Autodesk Inventor part; units mm, degrees
ref_plane "YZ Plane" through (0, 0, 0) normal (1, 0, 0) x (0, 1, 0)
ref_plane "XZ Plane" through (0, 0, 0) normal (0, 1, 0) x (-1, 0, 0)
ref_plane "XY Plane" through (0, 0, 0) normal (0, 0, 1) x (1, 0, 0)
sketch "草图1" plane through (0, 0, 0) normal (1, 0, 0) x (0, 1, 0)
  line L0 (-7.0511, 44.9164) -> (14.9489, 44.9164)
  line L1 (59.1261, -96.2836) -> (10.702, 41.9164)
  line L2 (10.702, 41.9164) -> (-7.0511, 41.9164)
  line L3 (-7.0511, 41.9164) -> (-7.0511, 44.9164)
  line L4 (57.8575, -77.5428) -> (14.9489, 44.9164)
  line L5 (63.8448, -94.6302) -> (59.1261, -96.2836)
  line L6 (63.8448, -94.6302) -> (57.8575, -77.5428)
  line L7 (10.702, 41.9164) -> (10.702, 44.9164)
  line L8 (14.9489, 44.9164) -> (14.9489, 41.9164)
  point P0 (0, 0)
  dimension "d1" = 3
  dimension "d2" = 109.31
  dimension "d3" = 138.2
  dimension "d10" = 5
  dimension "d90" = 22
extrude "拉伸1" add sketch "草图1" along normal blind 74
sketch "草图4" plane through (0, 14.9489, 44.9164) normal (0, 0.9437433, 0.3306791) x (1, 0, 0)
  line L0 (74, 3) -> (0, 3)
  line L1 (0, 3) -> (0, 0)
  line L2 (0, 0) -> (74, 0)
  line L3 (74, 0) -> (74, 3)
  line L4 (0, 0) -> (74, 0)
  line L5 (74, 147.865) -> (74, 0)
  line L6 (0, 0) -> (0, 147.865)
  point P0 (0, 37.4463)
  point P1 (67.5, 129.877)
  point P2 (0, 129.877)
  dimension "d11" = 3
extrude "拉伸3" add sketch "草图4" along normal blind 13
sketch "草图5" plane through (74, 0, 0) normal (1, 0, 0) x (0, 0, -1)
  line L0 (-27.5984, 19.9574) -> (113.9631, 69.5592)
  line L1 (113.9631, 69.5592) -> (114.7237, 67.3886)
  line L2 (114.7237, 67.3886) -> (-26.8378, 17.7868)
  line L3 (-26.8378, 17.7868) -> (-27.5984, 19.9574)
  line L4 (94.6302, 63.8448) -> (-42.0852, 15.9409)
  line L5 (-42.0852, 15.9409) -> (-40.3206, 10.9047)
  point P0 (0, 0)
  point P1 (78.0607, 56.3152)
  dimension "d15" = 1
  dimension "d16" = 150
  dimension "d17" = 2.3
  dimension "d22" = 15
extrude "拉伸4" cut sketch "草图5" against normal blind 5
sketch "草图6" plane through (0, 0, 0) normal (-1, 0, 0) x (0, 0, 1)
  line L0 (-113.9631, 69.5592) -> (27.5984, 19.9574)
  line L1 (27.5984, 19.9574) -> (26.8378, 17.7868)
  line L2 (26.8378, 17.7868) -> (-114.7237, 67.3886)
  line L3 (-114.7237, 67.3886) -> (-113.9631, 69.5592)
  line L4 (42.0852, 15.9409) -> (-94.6302, 63.8448)
  line L5 (42.0852, 15.9409) -> (38.373, 5.3464)
  point P0 (0, 0)
  point P1 (-78.0607, 56.3152)
  dimension "d20" = 1
  dimension "d21" = 2.3
  dimension "d23" = 15
  dimension "d24" = 150
extrude "拉伸5" cut sketch "草图6" against normal blind 5
sketch "草图8" plane through (74, 0, 0) normal (1, 0, 0) x (0, 0, -1)
  line L0 (96.2836, 59.1261) -> (95.7214, 60.7304)
  line L1 (95.7214, 60.7304) -> (76.8465, 54.1168)
  line L2 (76.8465, 54.1168) -> (77.4087, 52.5125)
  line L3 (77.4087, 52.5125) -> (96.2836, 59.1261)
  line L4 (96.2836, 59.1261) -> (95.7214, 60.7304)
  line L5 (-41.9164, 10.702) -> (96.2836, 59.1261)
  line L6 (95.7214, 60.7304) -> (-26.8378, 17.7868)
  point P0 (0, 0)
  point P1 (84.6027, 53.1652)
  dimension "d32" = 20
extrude "拉伸7" cut sketch "草图8" against normal blind 100
sketch "草图9" plane through (0, -7.0511, 44.9164) normal (0, 0, 1) x (1, 0, 0)
  line L0 (-3, 22) -> (77, 22)
  line L1 (77, 22) -> (77, 0)
  line L2 (77, 0) -> (-3, 0)
  line L3 (-3, 0) -> (-3, 22)
  line L4 (0, 22) -> (74, 22)
  line L5 (0, 0) -> (74, 0)
  line L6 (0, 0) -> (0, 22)
  line L7 (74, 22) -> (74, 0)
  point P0 (0, 7.0511)
  dimension "d35" = 3
  dimension "d36" = 3
extrude "拉伸8" add sketch "草图9" against normal blind 3 contours L0 L6 L2 L3 | L0 L1 L2 L7
sketch "草图10" plane through (74, 10.702, 41.9164) normal (0, 0, -1) x (-1, 0, 0)
  line L0 (10, -16.2531) -> (64, -16.2531)
  line L1 (64, -16.2531) -> (64, -17.7531)
  line L2 (64, -17.7531) -> (10, -17.7531)
  line L3 (10, -17.7531) -> (10, -16.2531)
  line L4 (-3, -17.7531) -> (77, -17.7531)
  line L5 (0, 0) -> (0, 41.8104)
  line L6 (77, -17.7531) -> (77, 4.2469)
  line L7 (74, 41.8104) -> (74, 0)
  point P0 (74, -10.702)
  point P1 (0, 38.8623)
  point P2 (67.5, 38.8623)
  point P3 (80, 48.424)
  dimension "d39" = 1.5
  dimension "d40" = 10
  dimension "d55" = 10
extrude "拉伸9" add sketch "草图10" along normal blind 10
sketch "草图11" plane through (-3, -7.0511, 44.9164) normal (0, -1, 0) x (1, 0, 0)
  line L0 (77, -3) -> (77, -122.3251)
  line L1 (3, -122.3251) -> (3, -3)
  line L2 (0, 0) -> (80, 0)
  line L3 (80, -3) -> (67, -3)
  line L4 (13, -3) -> (13, -13)
  line L5 (67, -13) -> (13, -13)
  point P0 (3, -44.9164)
  point P1 (59, -7)
  point P2 (21, -7)
  point P3 (70.75, -123.9692)
  point P4 (3.25, -123.9692)
  point P5 (3.25, -141.2)
  dimension "d44" = 18
  dimension "d45" = 18
  dimension "d53" = 7
  dimension "d54" = 7
  dimension "d56" = 3
  dimension "d57" = 8
  dimension "d58" = 6
hole "孔1" at (56, -7.0511, 37.9164) at (18, -7.0511, 37.9164) direction (0, 1, 0) diameter 2.013 depth 2 tip angle 118
sketch "草图21" plane through (74, 0, 0) normal (1, 0, 0) x (0, 0, -1)
  line L0 (-42.0852, 15.9409) -> (94.6302, 63.8448)
  line L1 (94.6302, 63.8448) -> (95.8266, 63.8448)
  line L2 (95.8266, 63.8448) -> (95.8266, 58.5781)
  line L3 (95.8266, 58.5781) -> (94.6302, 58.5781)
  line L4 (94.6302, 58.5781) -> (94.6302, 63.8448)
  point P0 (0, 0)
extrude "拉伸14" cut sketch "草图21" against normal blind 150
sketch "草图22" plane through (0, 10.702, 41.9164) normal (0, -0.9437433, -0.3306791) x (1, 0, 0)
  line L0 (5, -145.2818) -> (69, -145.2818)
  line L1 (64, -10.7184) -> (10, -10.7184)
  line L2 (10, -10.7184) -> (10, -145.2818)
  line L3 (10, -145.2818) -> (64, -145.2818)
  line L4 (64, -145.2818) -> (64, -10.7184)
  line L5 (74, 0) -> (74, -126.4381)
  line L6 (0, -126.4381) -> (0, 0)
  line L7 (74, -16.5731) -> (74, -146.0877)
  line L8 (69, -145.2818) -> (69, -146.0877)
  point P0 (0, -36.0194)
  point P1 (67.5, -127.0584)
  point P2 (0, -127.0584)
  point P3 (74, -146.0877)
  point P4 (64, -145.2818)
  point P5 (80, -133.0485)
  point P6 (0, -133.0485)
  point P7 (12, -145.2818)
  point P8 (0, -146.4381)
  point P9 (64, -145.2818)
  dimension "d74" = 10
  dimension "d75" = 10
  dimension "d76" = 5
extrude "拉伸15" cut sketch "草图22" against normal blind 2.5
sketch "草图25" plane through (0, 10.702, 41.9164) normal (0, -0.9437433, -0.3306791) x (1, 0, 0)
  line L0 (0, -126.4381) -> (0, 0)
  line L1 (69.9045, -127.7568) -> (0, -127.7568)
  line L2 (0, -127.7568) -> (0, -133.0485)
  line L3 (0, -133.0485) -> (69.9045, -133.0485)
  line L4 (69.9045, -133.0485) -> (69.9045, -127.7568)
  point P0 (0, -36.0194)
  point P1 (0, -127.7568)
extrude "拉伸16" cut sketch "草图25" against normal blind 1.7
properties part number "cover"
Here's how the part is built. I have some questions about the finished solid (model axes, mm). A direction names the side the tool comes from. Coordinates: 2 decimals unless noted, no trailing zeros. Order: outer loops, then holes, each group sorted by start corner. A loop starts at its lowest first (then second) coordinate and runs counter-clockwise, first axis right, second up. Notation, with made-up numbers: (-19.5, 12) -> (23.5, 12) arc R27 ccw to (23.5, 29) -> close; hole circle Ø10 at (9.25, 3). An arc over 180 degrees is marked (long way). Return JSON: item names as keys, results as strings.
1) If we section it at C-C on y = 5: List the corners of the cut face in (x, z) for me.
Conclusion:
{"outline": "(-3, 41.92) -> (77, 41.92) -> (77, 44.92) -> (-3, 44.92) -> close"}
2) If we section it at D-D on x = 24: List the corners of the cut face in (y, z) for me, plus the area to 3 significant figures.
Conclusion:
{"outline": "(-7.05, 31.92) -> (-5.55, 31.92) -> (-5.55, 41.92) -> (10.7, 41.92) -> (14.25, 31.8) -> (16.61, 32.63) -> (61.1, -94.36) -> (60.35, -94.63) -> (63.84, -94.63) -> (57.86, -77.54) -> (15.94, 42.09) -> (28.21, 46.38) -> (27.22, 49.22) -> (14.95, 44.92) -> (-7.05, 44.92) -> close", "area": "509 mm²"}
3) If we section it at B-B on z = -51.5: List the corners of the cut face in (x, y) for me.
Conclusion:
{"outline": "(0, 43.43) -> (10, 43.43) -> (10, 46.09) -> (64, 46.09) -> (64, 43.43) -> (74, 43.43) -> (74, 45.24) -> (69, 45.24) -> (69, 47.67) -> (74, 47.67) -> (74, 48.73) -> (0, 48.73) -> (0, 47.67) -> (5, 47.67) -> (5, 45.24) -> (0, 45.24) -> close"}
4) Thinking about a two-plate mould opening in Z: for faces 4 (the flat face through (66.465, 55.417, -80.552)), 5 (the flat face through (74, 30, -10)), 6 (the flat face through (5, 42, -38)), which applies, +Z half, -Z half, draft (parallel to the pull), parting line (faces both ways), or undercut?
Conclusion:
{"face 4": "-Z half", "face 5": "draft", "face 6": "undercut"}
5) On a 3-axis mill with a long thin cutter (end or side, diameter ignored), from which of +Z, -Z, +X, -X, +Y, -Y can I reach the whole of each face in a straight line? I mean faces 1 (the flat face through (75, 14.949, 43)), 2 (the flat face through (9.42, 30.16, -13.61)), 3 (the flat face through (69, 40, -33)). Say none if no direction works.
Conclusion:
{"face 1": "+Z, -Z, +X, +Y", "face 2": "-Z, +X, -X", "face 3": "+X"}
6) I'm going to push flat-ended pins straight in: P1, Ø14, axis at y = 27, z = -4.5, coming from the +X side; P2, Ø17.5, axis at x = 56.5, y = 8, coming from the -Z side; P3, Ø0.8, axis at y = -6.5, z = 37.5, coming from the -X side. Where does each tip first touch, or does it pass through?
Conclusion:
{"P1": "stops at x = 74", "P2": "stops at z = 31.8", "P3": "stops at x = 10"}
7) If we section it at A-A on x = 70.5: List the corners of the cut face in (y, z) for me.
Conclusion:
{"outline": "(-7.05, 41.92) -> (10.7, 41.92) -> (52.51, -77.41) -> (54.12, -76.85) -> (17.79, 26.84) -> (19.96, 27.6) -> (62.79, -94.63) -> (63.84, -94.63) -> (57.86, -77.54) -> (15.94, 42.09) -> (28.21, 46.38) -> (27.22, 49.22) -> (14.95, 44.92) -> (-7.05, 44.92) -> close"}
8) If I drill on probe 1 along Z at (x, y) = (18, -6.05); probe 2 along X at (y, z) = (55.5, -80); probe 3 along Y at (x, z) = (3, -73.5), over which ranges is the centre line in solid material (lowest first)?
Conclusion:
{"probe 1": "z = 31.92 to 36.91, 38.92 to 44.92", "probe 2": "x = 5 to 10, 64 to 69", "probe 3": "y = 51.14 to 52.94, 55.38 to 56.44"}
